```python
from build123d import *

# Parameters (mm, degrees)
F0_W         = 100
F0_H         = 100
F1_DEPTH     = 100
F2_R         = 5.08
F3_R         = 5.08
F4_T1_DEPTH  = 120.32
F4_T3_DEPTH  = 120.32
F5_T1_DEPTH  = 89.84
F5_S5_W      = 5.08
F5_S5_H      = 5.08
F5_T6_DEPTH  = 5.08
F5_S11_W     = 5.08
F5_S11_H     = 5.08
F5_T12_DEPTH = 5.08
F8_DEPTH     = 10
F10_R        = 8.3
F11_DEPTH    = 10
F12_R        = 8.3
F13_DEPTH    = 10
F9_R         = 8.3
F14_DEPTH    = 10
F15_R        = 8.3
F16_DEPTH    = 10
F17_R        = 8.3
F18_DEPTH    = 10


# Not quite as in the source:
# - a fillet or chamfer that OpenCascade refuses, or shapes differently, is made with other operations: its cross-section is extruded or revolved along the edge and cut away or added


with BuildPart() as f1:
    # F0 (on Top) → F1 (new body)
    with BuildSketch(Plane.XY):
        with Locations((-11.9530703868, 12.5334430486)):
            Rectangle(F0_W, F0_H)
    extrude(amount=F1_DEPTH)

    # F2
    f2_edges = [f1.edges().sort_by_distance(p)[0] for p in [
        (-11.95307, -37.466557, 100),
    ]]
    fillet(f2_edges, radius=F2_R)

    # F3
    f3_edges = [f1.edges().sort_by_distance(p)[0] for p in [
        (-11.95307, -37.466557, 0),
        (38.04693, -37.466557, 47.46),
        (-61.95307, -37.466557, 47.46),
        (-11.95307, 62.533443, 100),
        (-61.95307, 15.073443, 100),
        (38.04693, 15.073443, 100),
        (38.04693, 12.533443, 0),
        (38.04693, 62.533443, 50),
    ]]
    fillet(f3_edges, radius=F3_R)

    # F4: fillet of radius 5.08 on 4 edges, made by hand

    # F4_s2 → F4_t1 (cut)
    with BuildSketch(Plane.YZ.offset(-74.6530703868)):
        with BuildLine():
            ThreePointArc((57.4534430486, 0), (61.045545497, 1.4878975516), (62.5334430486, 5.08))
            Line((62.5334430486, 5.08), (62.5334430486, 0))
            Line((62.5334430486, 0), (57.4534430486, 0))
        make_face()
    extrude(amount=F4_T1_DEPTH, mode=Mode.SUBTRACT)

    # F4_s4 → F4_t3 (cut)
    with BuildSketch(Plane.XZ.offset(-75.2334430486)):
        with BuildLine():
            ThreePointArc((-61.9530703868, 5.08), (-60.4651728352, 1.4878975516), (-56.8730703868, 0))
            Line((-56.8730703868, 0), (-61.9530703868, 0))
            Line((-61.9530703868, 0), (-61.9530703868, 5.08))
        make_face()
    extrude(amount=F4_T3_DEPTH, mode=Mode.SUBTRACT)

    # F5: fillet of radius 5.08 on 1 edges, made by hand

    # F5_s2 → F5_t1 (cut)
    with BuildSketch(Plane.XY.offset(5.08)):
        with BuildLine():
            ThreePointArc((-61.9530703868, 57.4534430486), (-60.4651728352, 61.045545497), (-56.8730703868, 62.5334430486))
            Line((-56.8730703868, 62.5334430486), (-61.9530703868, 62.5334430486))
            Line((-61.9530703868, 62.5334430486), (-61.9530703868, 57.4534430486))
        make_face()
    extrude(amount=F5_T1_DEPTH, mode=Mode.SUBTRACT)


with BuildPart() as f5_tool4:
    # F5_s5 → F5_t6 (new body)
    with BuildSketch(Plane.YZ.offset(-56.8730703868)):
        with Locations((59.9934430486, 2.54)):
            Rectangle(F5_S5_W, F5_S5_H)
    extrude(amount=-F5_T6_DEPTH)

    # F5_s7 → F5_t8 (revolve, cut)
    with BuildSketch(Plane(origin=(-56.8730703868, 57.4534430486, 5.08), x_dir=(0, -0.7071067812, 0.7071067812), z_dir=(0, -0.7071067812, -0.7071067812))):
        with BuildLine():
            ThreePointArc((0, -5.08), (5.08, 0), (0, 5.08))
            Line((0, 5.08), (0, -5.08))
        make_face()
    revolve(axis=Axis((-56.8730703868, 57.4534430486, 5.08), (-1, 0, 0)), mode=Mode.SUBTRACT)


with BuildPart() as f1_1:
    add(f1.part)

    # F5_t3: cut F5_tool4
    add(f5_tool4.part, mode=Mode.SUBTRACT)


with BuildPart() as f5_tool10:
    # F5_s11 → F5_t12 (new body)
    with BuildSketch(Plane.YZ.offset(-56.8730703868)):
        with Locations((59.9934430486, 97.46)):
            Rectangle(F5_S11_W, F5_S11_H)
    extrude(amount=-F5_T12_DEPTH)

    # F5_s13 → F5_t14 (revolve, cut)
    with BuildSketch(Plane(origin=(-56.8730703868, 57.4534430486, 94.92), x_dir=(0, -0.7071067812, -0.7071067812), z_dir=(0, 0.7071067812, -0.7071067812))):
        with BuildLine():
            ThreePointArc((0, -5.08), (5.08, 0), (0, 5.08))
            Line((0, 5.08), (0, -5.08))
        make_face()
    revolve(axis=Axis((-56.8730703868, 57.4534430486, 94.92), (-1, 0, 0)), mode=Mode.SUBTRACT)


with BuildPart() as f1_2:
    add(f1_1.part)

    # F5_t9: cut F5_tool10
    add(f5_tool10.part, mode=Mode.SUBTRACT)

    # F7 (on face) → F8 (cut)
    with BuildSketch(Plane.XY.offset(100)):
        with BuildLine():
            Line((-11.9530703868, 12.5334430486), (-11.9530703868, 21.0658373489))
            ThreePointArc((-11.9530703868, 21.0658373489), (-17.9663578599, 18.5867909487), (-20.3459117026, 12.5334430486))
            Line((-20.3459117026, 12.5334430486), (-11.9530703868, 12.5334430486))
        make_face()
        with BuildLine():
            ThreePointArc((-20.3459117026, 12.5334430486), (-11.932694522, 4.4672112942), (-3.7491813868, 12.7663938329))
            ThreePointArc((-3.7491813868, 12.7663938329), (-6.1463125377, 18.601300803), (-11.9530703868, 21.0658373489))
            Line((-11.9530703868, 21.0658373489), (-11.9530703868, 12.5334430486))
            Line((-11.9530703868, 12.5334430486), (-20.3459117026, 12.5334430486))
        make_face()
    extrude(amount=-F8_DEPTH, mode=Mode.SUBTRACT)

    # F10 (on face) → F11 (cut)
    with BuildSketch(Plane(origin=(0, 62.5334430486, 0), x_dir=(-1, 0, 0), z_dir=(0, 1, 0))):
        with Locations((-10.5468751863, 50)):
            Circle(F10_R)
        with Locations((33.9843742549, 50)):
            Circle(F10_R)
    extrude(amount=-F11_DEPTH, mode=Mode.SUBTRACT)

    # F12 (on face) → F13 (cut)
    with BuildSketch(Plane(origin=(0, 0, 0), x_dir=(1, 0, 0), z_dir=(0, 0, -1))):
        with Locations((-26.988836811, 2.8129873745)):
            Circle(F12_R)
        with Locations((2.9531012963, 2.62785203)):
            Circle(F12_R)
        with Locations((3.9886479591, -28.1644973956)):
            Circle(F12_R)
        with Locations((-27.8392481293, -28.1644973956)):
            Circle(F12_R)
    extrude(amount=-F13_DEPTH, mode=Mode.SUBTRACT)

    # F9 (on face) → F14 (cut)
    with BuildSketch(Plane(origin=(-61.9530703868, 0, 0), x_dir=(0, -1, 0), z_dir=(-1, 0, 0))):
        with Locations((-27.5969797745, 65.0635367259)):
            Circle(F9_R)
        with Locations((-12.5334430486, 50)):
            Circle(F9_R)
        with Locations((2.3449583328, 64.8784013814)):
            Circle(F9_R)
        with Locations((3.3805049956, 34.0860519558)):
            Circle(F9_R)
        with Locations((-28.4473910928, 34.0860519558)):
            Circle(F9_R)
    extrude(amount=-F14_DEPTH, mode=Mode.SUBTRACT)

    # F15 (on face) → F16 (cut)
    with BuildSketch(Plane.YZ.offset(38.0469296132)):
        with Locations((26.2256339981, 36.3078090505)):
            Circle(F15_R)
        with Locations((12.5333450089, 50.0000980397)):
            Circle(F15_R)
        with Locations((-1.261167958, 63.7946110066)):
            Circle(F15_R)
    extrude(amount=-F16_DEPTH, mode=Mode.SUBTRACT)

    # F17 (on face) → F18 (cut)
    with BuildSketch(Plane.XZ.offset(37.4665569514)):
        with Locations((10.5468751863, 27.499999851)):
            Circle(F17_R)
        with Locations((10.5468751863, 72.4999979138)):
            Circle(F17_R)
        with Locations((-34.4531275332, 72.4999979138)):
            Circle(F17_R)
        with Locations((-34.4531275332, 27.499999851)):
            Circle(F17_R)
    extrude(amount=-F18_DEPTH, mode=Mode.SUBTRACT)


solid = f1_2.part
```
Model file for the job. Use its own axes, mm. A direction names the side the tool comes from. Give positions to 0.01 mm unless a question says otherwise; leave off trailing zeros. Write each loop counter-clockwise with the first axis right and the second up, starting at its lowest first coordinate (ties: lowest second). Pieces come first, ordered by that corner, then holes. Notation, with made-up numbers: (-11.5, 29.25) -> (-4.5, 29.25) arc R20 cw to (-4.5, 51.25) -> close; hole circle Ø8 at (42.5, -4). An arc over 180 degrees is marked (long way). Use CSV: the item, a comma, the result in double quotes. Start each with the question number.
1) Cut at C-C on z = 24. List the corners of the cut face in (x, y), plus the area to 3 significant figures.
2) Cut at B-B on x = -15.5. List the corners of the cut face in (y, z).
3) Tool access for faces 5 (the flat face through (-13, 13, 0)), 6 (the flat face through (-35, -27.467, 73)), 7 (the flat face through (-51.953, 29, 34)), 8 (the cylindrical face through (2.908, 19.935, 4.93)), 9 (the flat face through (-13, -37.467, 49)): list every direction of +Z, -Z, +X, -X, +Y, -Y with a clear straight run to the whole face (end or side of a thin tool).
4) Two-plate mould, pull along X, no slides. Class faces 1 (the cylindrical face through (33.117, 3.201, 70.793)), 2 (the flat face through (-51.953, 28, 65)), 3 (the cylindrical face through (36.52, -36.02, 50.63)), 4 (the cylindrical face through (-19.923, 25.671, 4.93)): released by +X, released by -X, zero draft, split by the parting line, or undercut.
5) Drill centre lines: L1, parallel to Z at x = 13.5, y = -29; L2, parallel to Y at x = -33.5, z = 31.5; L3, parallel to X at y = 2, z = 67.5. Where is each one in solid material? Low to high.
6) Cut at D-D on y = 16.5. List the corners of the cut face in (x, z), plus the area to 3 significant figures.
7) Cut at A-A on y = 2. List the corners of the cut face in (x, z), plus the area to 3 significant figures.
8) Pin check, flat tips, straight feed: P1, Ø5, axis at y = 30.5, z = 66.5, coming from the -X side; P2, Ø13.5, axis at x = 14.5, z = 54, coming from the +Y side; P3, Ø10, axis at x = 3.99, y = 28.16, coming from the -Z side; P4, Ø8.5, axis at x = -33, z = 53, coming from the +Y side. Stop position of each tip, or through.
Final values:
1,outline,"(-61.95, -32.39) arc R5.08 ccw to (-56.87, -37.47) -> (-41.98, -37.47) -> (-41.98, -27.47) -> (-26.93, -27.47) -> (-26.93, -37.47) -> (3.02, -37.47) -> (3.02, -27.47) -> (18.07, -27.47) -> (18.07, -37.47) -> (32.97, -37.47) arc R5.08 ccw to (38.05, -32.39) -> (38.05, 57.45) arc R5.08 ccw to (32.97, 62.53) -> (-56.87, 62.53) arc R5.08 ccw to (-61.95, 57.45) -> close"
1,area,"9,680 mm2"
2,outline,"(-37.47, 5.08) arc R5.08 ccw to (-32.39, 0) -> (57.45, 0) arc R5.08 ccw to (62.53, 5.08) -> (62.53, 94.92) arc R5.08 ccw to (57.45, 100) -> (20.32, 100) -> (20.32, 90) -> (5.22, 90) -> (5.22, 100) -> (-32.39, 100) arc R5.08 ccw to (-37.47, 94.92) -> close"
3,face 5,"-Z, +X, -X, +Y, -Y"
3,face 6,"-Y"
3,face 7,"-X"
3,face 8,"-Z"
3,face 9,"+Z, -Z, +X, -X, -Y"
4,face 1,"zero draft"
4,face 2,"released by -X"
4,face 3,"released by +X"
4,face 4,"undercut"
5,L1,"z = 0 to 19.74, 35.26 to 64.74, 80.26 to 100"
5,L2,"y = -27.47 to 62.53"
5,L3,"x = -51.95 to 28.05"
6,outline,"(-61.95, 5.08) arc R5.08 ccw to (-56.87, 0) -> (32.97, 0) arc R5.08 ccw to (38.05, 5.08) -> (38.05, 42.71) -> (28.05, 42.71) -> (28.05, 57.29) -> (38.05, 57.29) -> (38.05, 94.92) arc R5.08 ccw to (32.97, 100) -> (-4.64, 100) -> (-4.64, 90) -> (-19.46, 90) -> (-19.46, 100) -> (-56.87, 100) arc R5.08 ccw to (-61.95, 94.92) -> (-61.95, 57.29) -> (-51.95, 57.29) -> (-51.95, 42.71) -> (-61.95, 42.71) -> close"
6,area,"9,540 mm2"
7,outline,"(-61.95, 5.08) arc R5.08 ccw to (-56.87, 0) -> (-33.75, 0) -> (-33.75, 10) -> (-20.23, 10) -> (-20.23, 0) -> (-3.94, 0) -> (-3.94, 10) -> (9.84, 10) -> (9.84, 0) -> (32.97, 0) arc R5.08 ccw to (38.05, 5.08) -> (38.05, 56.16) -> (28.05, 56.16) -> (28.05, 71.43) -> (38.05, 71.43) -> (38.05, 94.92) arc R5.08 ccw to (32.97, 100) -> (-56.87, 100) arc R5.08 ccw to (-61.95, 94.92) -> (-61.95, 71.95) -> (-51.95, 71.95) -> (-51.95, 57.81) -> (-61.95, 57.81) -> (-61.95, 40.41) -> (-51.95, 40.41) -> (-51.95, 27.77) -> (-61.95, 27.77) -> close"
7,area,"9,280 mm2"
8,P1,"stops at x = -51.95"
8,P2,"stops at y = 62.53"
8,P3,"stops at z = 10"
8,P4,"stops at y = 52.53"
